Read the model definition and answer for the solid it produces. Units are mm, in the model's axes. A direction names the side the tool comes from. Give positions to 0.01 mm unless a question says otherwise; leave off trailing zeros. Order: outer loops, then holes, each group sorted by start corner. A loop starts at its lowest first (then second) coordinate and runs counter-clockwise, first axis right, second up. Notation, with made-up numbers: (12.5, 26) -> (42.5, 26) arc R26 ccw to (42.5, 55) -> close; hole circle Ø3 at (66, 19). An arc over 180 degrees is marked (long way). One line per question, with ' | ' between items. Start each with the question number.
```python
from build123d import *

# Parameters (mm, degrees)
SKETCH1_R           = 175
BOSS_EXTRUDE1_DEPTH = 10
SKETCH3_R           = 10
SKETCH3_W           = 162
SKETCH3_H           = 50
SKETCH3_W_2         = 175
SKETCH3_H_2         = 42.297309852
CUT_EXTRUDE2_DEPTH  = 10
CUT_EXTRUDE3_DEPTH  = 10
BOSS_EXTRUDE2_START = -75
SKETCH5_R           = 177
SKETCH5_R_2         = 175
BOSS_EXTRUDE2_DEPTH = 75


with BuildPart() as part:
    # Sketch1 → Boss-Extrude1 (new body)
    with BuildSketch(Plane(origin=(0, 0, 0), x_dir=(1, 0, 0), z_dir=(0, 1, 0))):
        with Locations(Location((0, 0, 0), (0, 0, 270))):
            Circle(SKETCH1_R)
    extrude(amount=BOSS_EXTRUDE1_DEPTH)

    # Sketch3 → Cut-Extrude2 (cut)
    with BuildSketch(Plane.XZ):
        with Locations(Location((-117.665653332, 106.704862813, 0), (0, 0, 270))):
            Circle(SKETCH3_R)
        with Locations(Location((117.665653332, 106.704862813, 0), (0, 0, 270))):
            Circle(SKETCH3_R)
        with Locations(Location((151.426262726, -48.693236313, 0), (0, 0, 270))):
            Circle(SKETCH3_R)
        with Locations(Location((-151.426262726, -48.693236313, 0), (0, 0, 270))):
            Circle(SKETCH3_R)
        with Locations((-0.423800225, -2.37885536)):
            Rectangle(SKETCH3_W, SKETCH3_H)
        with Locations((0, 119.225084577)):
            Rectangle(SKETCH3_W_2, SKETCH3_H_2)
    extrude(amount=-CUT_EXTRUDE2_DEPTH, mode=Mode.SUBTRACT)

    # Sketch4 → Cut-Extrude3 (cut)
    with BuildSketch(Plane.XZ):
        with BuildLine():
            Line((-14.298045865, -66.747113031), (14.298045865, -66.747113031))
            ThreePointArc((14.298045865, -66.747113031), (17.831426019, -68.210687012), (19.295, -71.744067166))
            Line((19.295, -71.744067166), (19.295, -100.340158896))
            ThreePointArc((19.295, -100.340158896), (17.832240237, -103.873462582), (14.299305419, -105.337113031))
            Line((14.299305419, -105.337113031), (-14.298045712, -105.337113031))
            ThreePointArc((-14.298045712, -105.337113031), (-17.831350955, -103.874338314), (-19.295, -100.341395166))
            Line((-19.295, -100.341395166), (-19.295, -71.744067166))
            ThreePointArc((-19.295, -71.744067166), (-17.831426019, -68.210687012), (-14.298045865, -66.747113031))
        make_face()
    extrude(amount=-CUT_EXTRUDE3_DEPTH, mode=Mode.SUBTRACT)

    # Sketch5 → Boss-Extrude2 (add)
    with BuildSketch(Plane(origin=(0, 10, 0), x_dir=(1, 0, 0), z_dir=(0, 1, 0)).offset(BOSS_EXTRUDE2_START)):
        with Locations(Location((0, 0, 0), (0, 0, 270))):
            Circle(SKETCH5_R)
        with Locations(Location((0, 0, 0), (0, 0, 270))):
            Circle(SKETCH5_R_2, mode=Mode.SUBTRACT)
    extrude(amount=BOSS_EXTRUDE2_DEPTH)


solid = part.part
```
Q1. Find the intervals of material crossed by line 1 (Z direction, x = -2.5, y = -4.5); line 2 (X direction, y = -21, z = 0); line 3 (Z direction, x = 159, y = -1), in increasing order.
Q2. A cutting plane is placed at D-D, the plane y = -12.5. Determine the outline of the cut face in (x, z), then the cut area to 3 significant figures.
Q3. A cutting plane is placed at B-B, the plane z = 0. Determine the outline of the cut face in (x, y).
Q4. Given P1, Ø6, axis at x = 1.5, y = -21.5, coming from the +Z side; P2, Ø10, axis at x = 125, y = -28, coming from the +Z side; P3, Ø8, axis at y = 5, z = 6.5, coming from the +X side; P4, Ø8, axis at y = -53.5, z = 88.5, coming from the -X side, each flat-ended and moving along its own axis, determine where each tip first touches the part or whether it passes through.
Q5. Determine the mould class of faces 4 (the flat face through (171, -65, -40)), 5 (the cylindrical face through (-121.5, 4.93, 97.47)), 6 (the cylindrical face through (-172.79, -28.02, -38.37)), 7 (the flat face through (80.576, 5, -3)) for opening direction X: pulls with the +X half, pulls with the -X half, needs draft (parallel to the pull), parting line crosses it, or undercut.
Q6. Which of the six approach directions +Z, -Z, +X, -X, +Y, -Y give full straight-line access (tool end or side, diameter ignored) to faces 1 (the cylindrical face through (173.51, -32.96, -22.78)), 2 (the flat face through (87.5, 5, 119)), 3 (the flat face through (2, 10, -42))?
Q7. A cutting plane is placed at A-A, the plane x = 0. Determine the outline of the cut face in (y, z).
Q8. A cutting plane is placed at C-C, the plane z = -46. Determine the outline of the cut face in (x, y).
Geometry results:
1) line 1: -176.98 to -174.98, 174.98 to 176.98 | line 2: -177 to -175, 175 to 177 | line 3: -77.77 to -73.1, 73.1 to 77.77
2) outline: circle Ø354 at (0, 0); hole circle Ø350 at (0, 0) | area: 2,210 mm²
3) outline: (-177, -65) -> (-175, -65) -> (-175, 0) -> (-81.42, 0) -> (-81.42, 10) -> (-177, 10) -> close; (80.58, 0) -> (175, 0) -> (175, -65) -> (177, -65) -> (177, 10) -> (80.58, 10) -> close
4) P1: z = 177 | P2: z = 130.11 | P3: x = 176.98 | P4: x = -155.53
5) face 4: needs draft | face 5: undercut | face 6: parting line crosses it | face 7: undercut
6) face 1: -Y | face 2: +Y, -Y | face 3: +Z, -Z, +X, -X, +Y
7) outline: (-65, -177) -> (10, -177) -> (10, -105.34) -> (0, -105.34) -> (0, -175) -> (-65, -175) -> close; (-65, 175) -> (0, 175) -> (0, 140.37) -> (10, 140.37) -> (10, 177) -> (-65, 177) -> close; (0, -66.75) -> (10, -66.75) -> (10, -27.38) -> (0, -27.38) -> close; (0, 22.62) -> (10, 22.62) -> (10, 98.08) -> (0, 98.08) -> close
8) outline: (-170.92, -65) -> (-168.85, -65) -> (-168.85, 0) -> (-161.06, 0) -> (-161.06, 10) -> (-170.92, 10) -> close; (-141.8, 0) -> (141.8, 0) -> (141.8, 10) -> (-141.8, 10) -> close; (161.06, 0) -> (168.85, 0) -> (168.85, -65) -> (170.92, -65) -> (170.92, 10) -> (161.06, 10) -> close
